Input: part model. Units: mm. Frame: model coordinates. A direction names the side the tool comes from. Round coordinates to 2 decimals unless told otherwise and drop trailing zeros. Loops run counter-clockwise (first coordinate to the right, second up) from the corner with the lowest first, then second, coordinate; pieces in that order, holes last. Notation, with made-up numbers: M -11.5,-8 L 19.5,-8 A16 cw 19.5,14 Z; hole C 54,14.25 d5. An arc over 180 degrees is marked long. Use one line per item in the form item = value. Start each with the question number.
Q1. Section query A-A, the plane x = -14. Output: boundary loops of the cut face in (y, z).
Q2. Section query B-B, the plane y = 70. Output: boundary loops of the cut face in (x, z), and give its area (4 significant figures).
Q3. Section query D-D, the plane x = 20. Output: boundary loops of the cut face in (y, z).
Q4. Mould query, pull axis X, two halves, no side actions, for faces 6 (the flat face through (52.5, 42, 0)), 7 (the flat face through (50, 80, 20)), 8 (the flat face through (0, 62.5, 30)), 9 (the flat face through (-1, 84, 30)). Classes: pulls with the +X half, pulls with the -X half, needs draft (parallel to the pull), parting line crosses it, or undercut.
Q5. Access query for faces 1 (the flat face through (-7.5, 70, 30)), 2 (the flat face through (-4, 82.5, 29)), 3 (the flat face through (-1, 51, 32.5)), 4 (the flat face through (50, 65, 20)), 5 (the flat face through (-1, 0, 0)). Directions: +Z, -Z, +X, -X, +Y, -Y. A direction counts if a zero-diameter tool reaches every point of the face in a straight line with its end or side. Return the directions, or none.
Q6. First-contact query: P1, Ø3, axis at x = -39.5, z = 13.5, coming from the -Y side; P2, Ø4, axis at x = -11, z = -9, coming from the +Y side; P3, Ø6, axis at x = 22, y = 72.5, coming from the +Z side; P4, Ø1.5, axis at x = 8, z = 24.5, coming from the +Y side. Flat tips, straight axial feed; report the tip coordinate or a pass-through.
Q7. Section query C-C, the plane y = 53. Output: boundary loops of the cut face in (x, z).
Q8. Ray query, line 1 along Z through (x, y) = (31, 74.5); line 2 along X through (y, z) = (29, 27); line 3 along Y through (x, z) = (20, 29). Return the intervals inside material, ascending.
```python
from build123d import *

# Parameters (mm, degrees)
SKETCH1_W           = 105
SKETCH1_H           = 65
BOSS_EXTRUDE1_DEPTH = 5
BOSS_EXTRUDE2_DEPTH = 20
SKETCH3_W           = 105
SKETCH3_H           = 65
SKETCH3_W_2         = 95
SKETCH3_H_2         = 55
BOSS_EXTRUDE3_DEPTH = 60
SKETCH4_W           = 100
SKETCH4_H           = 60
CUT_EXTRUDE1_DEPTH  = 2.5
SKETCH5_W           = 15
SKETCH5_H           = 15
SKETCH5_R           = 7.5
CUT_EXTRUDE3_DEPTH  = 10
SKETCH6_W           = 15
SKETCH6_H           = 15
CUT_EXTRUDE4_DEPTH  = 10
BOSS_EXTRUDE4_DEPTH = 95


with BuildPart() as part:
    # Sketch1 → Boss-Extrude1 (new body)
    with BuildSketch(Plane(origin=(0, 0, 0), x_dir=(1, 0, 0), z_dir=(0, 1, 0))):
        Rectangle(SKETCH1_W, SKETCH1_H)
    extrude(amount=BOSS_EXTRUDE1_DEPTH)

    # Sketch2 → Boss-Extrude2 (add)
    with BuildSketch(Plane(origin=(0, 5, 0), x_dir=(1, 0, 0), z_dir=(0, 1, 0))):
        Polygon((-47.5, -32.5), (-47.5, 27.5), (47.5, 27.5), (47.5, -32.5), (52.5, -32.5), (52.5, 32.5), (-52.5, 32.5), (-52.5, -32.5), align=None)
    extrude(amount=BOSS_EXTRUDE2_DEPTH)

    # Sketch3 → Boss-Extrude3 (add)
    with BuildSketch(Plane(origin=(0, 25, 0), x_dir=(1, 0, 0), z_dir=(0, 1, 0))):
        Rectangle(SKETCH3_W, SKETCH3_H)
        Rectangle(SKETCH3_W_2, SKETCH3_H_2, mode=Mode.SUBTRACT)
    extrude(amount=BOSS_EXTRUDE3_DEPTH)

    # Sketch4 → Cut-Extrude1 (cut)
    with BuildSketch(Plane(origin=(0, 85, 0), x_dir=(1, 0, 0), z_dir=(0, 1, 0))):
        Rectangle(SKETCH4_W, SKETCH4_H)
    extrude(amount=-CUT_EXTRUDE1_DEPTH, mode=Mode.SUBTRACT)

    # Sketch5 → Cut-Extrude3 (cut)
    with BuildSketch(Plane.XY.offset(32.5)):
        with Locations((0, 70)):
            Rectangle(SKETCH5_W, SKETCH5_H)
        with Locations((20, 70)):
            Circle(SKETCH5_R)
    extrude(amount=-CUT_EXTRUDE3_DEPTH, mode=Mode.SUBTRACT)

    # Sketch6 → Cut-Extrude4 (cut)
    with BuildSketch(Plane(origin=(52.5, 0, 0), x_dir=(0, 0, -1), z_dir=(1, 0, 0))):
        with Locations((-20, 72.5)):
            Rectangle(SKETCH6_W, SKETCH6_H)
    extrude(amount=-CUT_EXTRUDE4_DEPTH, mode=Mode.SUBTRACT)

    # Sketch10 → Boss-Extrude4 (add)
    with BuildSketch(Plane(origin=(-47.5, 0, 0), x_dir=(0, 0, -1), z_dir=(1, 0, 0))):
        Polygon((-32.5, 5), (27.5, 27.267325642), (27.5, 5), align=None)
    extrude(amount=BOSS_EXTRUDE4_DEPTH)


solid = part.part
```
Results found:
q1.outline = M 0,-32.5 L 85,-32.5 L 85,-30 L 82.5,-30 L 82.5,-27.5 L 27.27,-27.5 L 5,32.5 L 0,32.5 Z; M 25,27.5 L 82.5,27.5 L 82.5,30 L 85,30 L 85,32.5 L 25,32.5 Z
q2.outline = M -52.5,-32.5 L 52.5,-32.5 L 52.5,12.5 L 47.5,12.5 L 47.5,-27.5 L -47.5,-27.5 L -47.5,27.5 L -7.5,27.5 L -7.5,32.5 L -52.5,32.5 Z; M 7.5,27.5 L 12.5,27.5 L 12.5,32.5 L 7.5,32.5 Z; M 27.5,27.5 L 52.5,27.5 L 52.5,32.5 L 27.5,32.5 Z
q2.area = 1,375 mm²
q3.outline = M 0,-32.5 L 85,-32.5 L 85,-30 L 82.5,-30 L 82.5,-27.5 L 27.27,-27.5 L 5,32.5 L 0,32.5 Z; M 25,27.5 L 62.5,27.5 L 62.5,32.5 L 25,32.5 Z; M 77.5,27.5 L 82.5,27.5 L 82.5,30 L 85,30 L 85,32.5 L 77.5,32.5 Z
q4.face_6 = pulls with the +X half
q4.face_7 = needs draft
q4.face_8 = undercut
q4.face_9 = undercut
q5.face_1 = +Z
q5.face_2 = +Y
q5.face_3 = +Z, +X, -X, +Y, -Y
q5.face_4 = +X
q5.face_5 = +Z, -Z, +X, -X, -Y
q6.P1 = 0
q6.P2 = 21.14
q6.P3 = -27.5
q6.P4 = 8.25
q7.outline = M -52.5,-32.5 L 52.5,-32.5 L 52.5,32.5 L -52.5,32.5 Z; hole M -47.5,-27.5 L 47.5,-27.5 L 47.5,27.5 L -47.5,27.5 Z
q8.line_1 = -32.5 to -27.5, 27.5 to 32.5
q8.line_2 = -52.5 to -47.5, 47.5 to 52.5
q8.line_3 = 0 to 6.3, 25 to 62.5, 77.5 to 82.5
